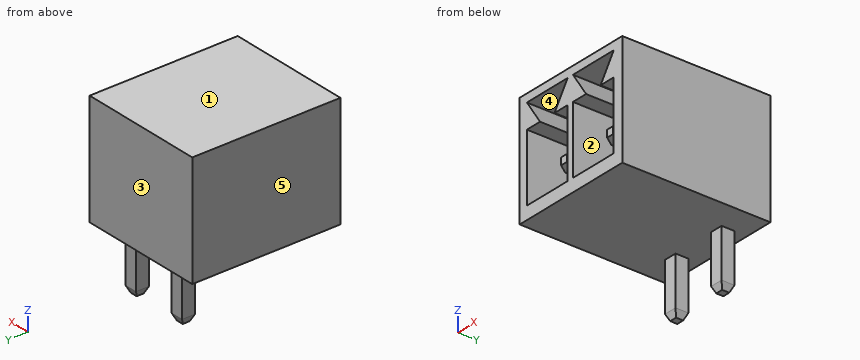
from build123d import *
from OCP.BRepFilletAPI import BRepFilletAPI_MakeChamfer

# Parameters (mm, degrees)
SKETCH_1_W                          = 7.8
SKETCH_1_H                          = 9.2
EXTRUDE_1_DEPTH                     = 7
SKETCH_2_W                          = 0.8
SKETCH_2_H                          = 0.8
EXTRUDE_2_DEPTH                     = 3.4
CHAMFER_1_SIZE                      = 0.4
CHAMFER_1_SIZE2                     = 0.178091474
CUT_EXTRUDE_1_DEPTH                 = 7
PATTERN_LINEAR_1_COUNT              = 3
PATTERN_LINEAR_1_PITCH              = 3.5
CHAMFER_1_OF_PATTERN_LINEAR_1_SIZE  = 0.4
CHAMFER_1_OF_PATTERN_LINEAR_1_SIZE2 = 0.178091474
PATTERN_LINEAR_2_COUNT              = 2
PATTERN_LINEAR_2_PITCH              = 3.5
SKETCH_4_W                          = 0.8
SKETCH_4_H                          = 0.8
EXTRUDE_3_DEPTH                     = 6
CHAMFER_2_SIZE                      = 0.4
CHAMFER_2_SIZE2                     = 0.178091474
PATTERN_LINEAR_3_COUNT              = 2
PATTERN_LINEAR_3_PITCH              = 3.5
CHAMFER_2_OF_PATTERN_LINEAR_3_SIZE  = 0.4
CHAMFER_2_OF_PATTERN_LINEAR_3_SIZE2 = 0.178091474


with BuildPart() as part:
    # Эскиз1 → Бобышка-Вытянуть1 (new body)
    with BuildSketch(Plane.XY):
        with Locations((0, 4.6)):
            Rectangle(SKETCH_1_W, SKETCH_1_H)
    extrude(amount=EXTRUDE_1_DEPTH)

    # Эскиз2 → Бобышка-Вытянуть2 (add)
    with BuildSketch(Plane(origin=(0, 0, 0), x_dir=(-1, 0, 0), z_dir=(0, 0, -1))):
        with Locations((-1.75, 8)):
            Rectangle(SKETCH_2_W, SKETCH_2_H)
    extrude_2 = extrude(amount=EXTRUDE_2_DEPTH)

    # Фаска1: one chamfer whose edges measure the first distance from different faces: ONE call of the kernel's chamfer builder (chamfer() names one face for all edges)
    chamfer_1_edges_1 = [part.edges().sort_by_distance(p)[0] for p in [
        (1.35, 8, -3.4),
    ]]
    chamfer_1_side_1 = [part.faces().sort_by_distance(p)[0] for p in [
        (1.35, 8, -1.7),
    ]]
    chamfer_1_edges_2 = [part.edges().sort_by_distance(p)[0] for p in [
        (1.75, 8.4, -3.4),
    ]]
    chamfer_1_side_2 = [part.faces().sort_by_distance(p)[0] for p in [
        (1.75, 8.4, -1.7),
    ]]
    chamfer_1_edges_3 = [part.edges().sort_by_distance(p)[0] for p in [
        (2.15, 8, -3.4),
    ]]
    chamfer_1_side_3 = [part.faces().sort_by_distance(p)[0] for p in [
        (2.15, 8, -1.7),
    ]]
    chamfer_1_edges_4 = [part.edges().sort_by_distance(p)[0] for p in [
        (1.75, 7.6, -3.4),
    ]]
    chamfer_1_side_4 = [part.faces().sort_by_distance(p)[0] for p in [
        (1.75, 7.6, -1.7),
    ]]
    chamfer_1 = BRepFilletAPI_MakeChamfer(part.part.solid().wrapped)
    for e in chamfer_1_edges_1:
        chamfer_1.Add(CHAMFER_1_SIZE, CHAMFER_1_SIZE2, e.wrapped, chamfer_1_side_1[0].wrapped)  # the first distance lies on this face
    for e in chamfer_1_edges_2:
        chamfer_1.Add(CHAMFER_1_SIZE, CHAMFER_1_SIZE2, e.wrapped, chamfer_1_side_2[0].wrapped)  # the first distance lies on this face
    for e in chamfer_1_edges_3:
        chamfer_1.Add(CHAMFER_1_SIZE, CHAMFER_1_SIZE2, e.wrapped, chamfer_1_side_3[0].wrapped)  # the first distance lies on this face
    for e in chamfer_1_edges_4:
        chamfer_1.Add(CHAMFER_1_SIZE, CHAMFER_1_SIZE2, e.wrapped, chamfer_1_side_4[0].wrapped)  # the first distance lies on this face
    add(Compound.cast(chamfer_1.Shape()), mode=Mode.REPLACE)

    # Эскиз3 → Вырез-Вытянуть1 (cut)
    with BuildSketch(Plane.XZ):
        Polygon((0.15, 0.8), (3.25, 0.8), (3.25, 5), (2.25, 5), (3.25, 6.5), (0.15, 6.5), (1.15, 5), (0.15, 5), align=None)
    cut_extrude_1 = extrude(amount=-CUT_EXTRUDE_1_DEPTH, mode=Mode.SUBTRACT)

    # Линейный массив1: Бобышка-Вытянуть2 ×3, 1 skipped
    with Locations(*[(-i * PATTERN_LINEAR_1_PITCH, 0, 0) for i in range(1, PATTERN_LINEAR_1_COUNT) if i not in (2,)]):
        add(extrude_2)

    # Фаска1 of Линейный массив1: one chamfer whose edges measure the first distance from different faces: ONE call of the kernel's chamfer builder (chamfer() names one face for all edges)
    chamfer_1_of_pattern_linear_1_edges_1 = [part.edges().sort_by_distance(p)[0] for p in [
        (-2.15, 8, -3.4),
    ]]
    chamfer_1_of_pattern_linear_1_side_1 = [part.faces().sort_by_distance(p)[0] for p in [
        (-2.15, 8, -1.7),
    ]]
    chamfer_1_of_pattern_linear_1_edges_2 = [part.edges().sort_by_distance(p)[0] for p in [
        (-1.75, 8.4, -3.4),
    ]]
    chamfer_1_of_pattern_linear_1_side_2 = [part.faces().sort_by_distance(p)[0] for p in [
        (-1.75, 8.4, -1.7),
    ]]
    chamfer_1_of_pattern_linear_1_edges_3 = [part.edges().sort_by_distance(p)[0] for p in [
        (-1.35, 8, -3.4),
    ]]
    chamfer_1_of_pattern_linear_1_side_3 = [part.faces().sort_by_distance(p)[0] for p in [
        (-1.35, 8, -1.7),
    ]]
    chamfer_1_of_pattern_linear_1_edges_4 = [part.edges().sort_by_distance(p)[0] for p in [
        (-1.75, 7.6, -3.4),
    ]]
    chamfer_1_of_pattern_linear_1_side_4 = [part.faces().sort_by_distance(p)[0] for p in [
        (-1.75, 7.6, -1.7),
    ]]
    chamfer_1_of_pattern_linear_1 = BRepFilletAPI_MakeChamfer(part.part.solid().wrapped)
    for e in chamfer_1_of_pattern_linear_1_edges_1:
        chamfer_1_of_pattern_linear_1.Add(CHAMFER_1_OF_PATTERN_LINEAR_1_SIZE, CHAMFER_1_OF_PATTERN_LINEAR_1_SIZE2, e.wrapped, chamfer_1_of_pattern_linear_1_side_1[0].wrapped)  # the first distance lies on this face
    for e in chamfer_1_of_pattern_linear_1_edges_2:
        chamfer_1_of_pattern_linear_1.Add(CHAMFER_1_OF_PATTERN_LINEAR_1_SIZE, CHAMFER_1_OF_PATTERN_LINEAR_1_SIZE2, e.wrapped, chamfer_1_of_pattern_linear_1_side_2[0].wrapped)  # the first distance lies on this face
    for e in chamfer_1_of_pattern_linear_1_edges_3:
        chamfer_1_of_pattern_linear_1.Add(CHAMFER_1_OF_PATTERN_LINEAR_1_SIZE, CHAMFER_1_OF_PATTERN_LINEAR_1_SIZE2, e.wrapped, chamfer_1_of_pattern_linear_1_side_3[0].wrapped)  # the first distance lies on this face
    for e in chamfer_1_of_pattern_linear_1_edges_4:
        chamfer_1_of_pattern_linear_1.Add(CHAMFER_1_OF_PATTERN_LINEAR_1_SIZE, CHAMFER_1_OF_PATTERN_LINEAR_1_SIZE2, e.wrapped, chamfer_1_of_pattern_linear_1_side_4[0].wrapped)  # the first distance lies on this face
    add(Compound.cast(chamfer_1_of_pattern_linear_1.Shape()), mode=Mode.REPLACE)

    # Линейный массив2: Вырез-Вытянуть1 ×2
    with Locations(*[(-i * PATTERN_LINEAR_2_PITCH, 0, 0) for i in range(1, PATTERN_LINEAR_2_COUNT)]):
        add(cut_extrude_1, mode=Mode.SUBTRACT)

    # Эскиз4 → Бобышка-Вытянуть3 (add)
    with BuildSketch(Plane.XZ.offset(-7)):
        with Locations((1.75, 3)):
            Rectangle(SKETCH_4_W, SKETCH_4_H)
    extrude_3 = extrude(amount=EXTRUDE_3_DEPTH)

    # Фаска2: one chamfer whose edges measure the first distance from different faces: ONE call of the kernel's chamfer builder (chamfer() names one face for all edges)
    chamfer_2_edges_1 = [part.edges().sort_by_distance(p)[0] for p in [
        (2.15, 1, 3),
    ]]
    chamfer_2_side_1 = [part.faces().sort_by_distance(p)[0] for p in [
        (2.15, 4, 3),
    ]]
    chamfer_2_edges_2 = [part.edges().sort_by_distance(p)[0] for p in [
        (1.75, 1, 3.4),
    ]]
    chamfer_2_side_2 = [part.faces().sort_by_distance(p)[0] for p in [
        (1.75, 4, 3.4),
    ]]
    chamfer_2_edges_3 = [part.edges().sort_by_distance(p)[0] for p in [
        (1.35, 1, 3),
    ]]
    chamfer_2_side_3 = [part.faces().sort_by_distance(p)[0] for p in [
        (1.35, 4, 3),
    ]]
    chamfer_2_edges_4 = [part.edges().sort_by_distance(p)[0] for p in [
        (1.75, 1, 2.6),
    ]]
    chamfer_2_side_4 = [part.faces().sort_by_distance(p)[0] for p in [
        (1.75, 4, 2.6),
    ]]
    chamfer_2 = BRepFilletAPI_MakeChamfer(part.part.solid().wrapped)
    for e in chamfer_2_edges_1:
        chamfer_2.Add(CHAMFER_2_SIZE, CHAMFER_2_SIZE2, e.wrapped, chamfer_2_side_1[0].wrapped)  # the first distance lies on this face
    for e in chamfer_2_edges_2:
        chamfer_2.Add(CHAMFER_2_SIZE, CHAMFER_2_SIZE2, e.wrapped, chamfer_2_side_2[0].wrapped)  # the first distance lies on this face
    for e in chamfer_2_edges_3:
        chamfer_2.Add(CHAMFER_2_SIZE, CHAMFER_2_SIZE2, e.wrapped, chamfer_2_side_3[0].wrapped)  # the first distance lies on this face
    for e in chamfer_2_edges_4:
        chamfer_2.Add(CHAMFER_2_SIZE, CHAMFER_2_SIZE2, e.wrapped, chamfer_2_side_4[0].wrapped)  # the first distance lies on this face
    add(Compound.cast(chamfer_2.Shape()), mode=Mode.REPLACE)

    # Линейный массив3: Бобышка-Вытянуть3 ×2
    with Locations(*[(-i * PATTERN_LINEAR_3_PITCH, 0, 0) for i in range(1, PATTERN_LINEAR_3_COUNT)]):
        add(extrude_3)

    # Фаска2 of Линейный массив3: one chamfer whose edges measure the first distance from different faces: ONE call of the kernel's chamfer builder (chamfer() names one face for all edges)
    chamfer_2_of_pattern_linear_3_edges_1 = [part.edges().sort_by_distance(p)[0] for p in [
        (-1.35, 1, 3),
    ]]
    chamfer_2_of_pattern_linear_3_side_1 = [part.faces().sort_by_distance(p)[0] for p in [
        (-1.35, 4, 3),
    ]]
    chamfer_2_of_pattern_linear_3_edges_2 = [part.edges().sort_by_distance(p)[0] for p in [
        (-1.75, 1, 3.4),
    ]]
    chamfer_2_of_pattern_linear_3_side_2 = [part.faces().sort_by_distance(p)[0] for p in [
        (-1.75, 4, 3.4),
    ]]
    chamfer_2_of_pattern_linear_3_edges_3 = [part.edges().sort_by_distance(p)[0] for p in [
        (-2.15, 1, 3),
    ]]
    chamfer_2_of_pattern_linear_3_side_3 = [part.faces().sort_by_distance(p)[0] for p in [
        (-2.15, 4, 3),
    ]]
    chamfer_2_of_pattern_linear_3_edges_4 = [part.edges().sort_by_distance(p)[0] for p in [
        (-1.75, 1, 2.6),
    ]]
    chamfer_2_of_pattern_linear_3_side_4 = [part.faces().sort_by_distance(p)[0] for p in [
        (-1.75, 4, 2.6),
    ]]
    chamfer_2_of_pattern_linear_3 = BRepFilletAPI_MakeChamfer(part.part.solid().wrapped)
    for e in chamfer_2_of_pattern_linear_3_edges_1:
        chamfer_2_of_pattern_linear_3.Add(CHAMFER_2_OF_PATTERN_LINEAR_3_SIZE, CHAMFER_2_OF_PATTERN_LINEAR_3_SIZE2, e.wrapped, chamfer_2_of_pattern_linear_3_side_1[0].wrapped)  # the first distance lies on this face
    for e in chamfer_2_of_pattern_linear_3_edges_2:
        chamfer_2_of_pattern_linear_3.Add(CHAMFER_2_OF_PATTERN_LINEAR_3_SIZE, CHAMFER_2_OF_PATTERN_LINEAR_3_SIZE2, e.wrapped, chamfer_2_of_pattern_linear_3_side_2[0].wrapped)  # the first distance lies on this face
    for e in chamfer_2_of_pattern_linear_3_edges_3:
        chamfer_2_of_pattern_linear_3.Add(CHAMFER_2_OF_PATTERN_LINEAR_3_SIZE, CHAMFER_2_OF_PATTERN_LINEAR_3_SIZE2, e.wrapped, chamfer_2_of_pattern_linear_3_side_3[0].wrapped)  # the first distance lies on this face
    for e in chamfer_2_of_pattern_linear_3_edges_4:
        chamfer_2_of_pattern_linear_3.Add(CHAMFER_2_OF_PATTERN_LINEAR_3_SIZE, CHAMFER_2_OF_PATTERN_LINEAR_3_SIZE2, e.wrapped, chamfer_2_of_pattern_linear_3_side_4[0].wrapped)  # the first distance lies on this face
    add(Compound.cast(chamfer_2_of_pattern_linear_3.Shape()), mode=Mode.REPLACE)


solid = part.part
Can you work these out from the model? Positions are in its coordinate system, mm. Face numbers are marked on the shaded views. A direction names the side the tool comes from. Coordinates: 2 decimals unless noted, no trailing zeros. Write each loop counter-clockwise with the first axis right and the second up, starting at its lowest first coordinate (ties: lowest second). Pieces come first, ordered by that corner, then holes. Notation, with made-up numbers: (56, 29.5) - (66, 29.5) arc R11 ccw to (66, 35.5) - close; hole circle Ø3 at (-27, 71.25). An arc over 180 degrees is marked (long way). Return JSON: item names as keys, results as strings. Group by question number.
Item 1: If we section it at A-A (y = 5.5): Write out the boundary of the cut face in (x, z), then the cut area to 3 significant figures.
Item 2: If we section it at C-C (x = -2.75): Write out the boundary of the cut face in (y, z), then the cut area to 3 significant figures.
Item 3: Which directions (+Z, -Z, +X, -X, +Y, -Y) give clear straight access to the entire face, cutting with the end or side of a thin tool? Please do the marked faces 4 and 5.
Item 4: Please list where these lines run through material, in increasing order: probe 1 along X at (y, z) = (4, 4.5); probe 2 along Z at (x, y) = (2, 5); probe 3 along X at (y, z) = (2, 5.5).
Item 5: If we section it at D-D (z = 1): Write out the boundary of the cut face in (x, y).
Item 6: We'd pull the mould along Z, two halves only. Please class the marked faces 1, 2 and 3: pulls with the +Z half, pulls with the -Z half, needs draft (parallel to the pull), parting line crosses it, or undercut.
Item 7: If we section it at B-B (z = -0.5): Write out the boundary of the cut face in (x, y), then the cut area to 3 significant figures.
Item 8: I'm going to push flat-ended pins straight in: pin 1 Ø0.6 at (x, y) = (-1.5, 3) entering from -Z; pin 2 Ø0.6 at (y, z) = (8, -2) entering from -X; pin 3 Ø0.5 at (x, z) = (1.5, 3) entering from -Y. Where does each tip first touch, or does it pass through?
Return value:
{
 "1": {"outline": "(-3.9, 0) - (3.9, 0) - (3.9, 7) - (-3.9, 7) - close; (-2.15, 2.6) - (-1.35, 2.6) - (-1.35, 3.4) - (-2.15, 3.4) - close; (1.35, 2.6) - (2.15, 2.6) - (2.15, 3.4) - (1.35, 3.4) - close; hole (-3.35, 0.8) - (-0.25, 0.8) - (-0.25, 5) - (-1.25, 5) - (-0.25, 6.5) - (-3.35, 6.5) - (-2.35, 5) - (-3.35, 5) - close; hole (0.15, 0.8) - (3.25, 0.8) - (3.25, 5) - (2.25, 5) - (3.25, 6.5) - (0.15, 6.5) - (1.15, 5) - (0.15, 5) - close", "area": "23.5 mm^2"},
 "2": {"outline": "(0, 0) - (9.2, 0) - (9.2, 7) - (0, 7) - (0, 6.5) - (7, 6.5) - (7, 5.6) - (0, 5.6) - (0, 5) - (7, 5) - (7, 0.8) - (0, 0.8) - close", "area": "28.7 mm^2"},
 "3": {"face 4": "-Y", "face 5": "+Z, -Z, -X, +Y, -Y"},
 "4": {"probe 1": "x = -3.9 to -3.35, -0.25 to 0.15, 3.25 to 3.9", "probe 2": "z = 0 to 0.8, 2.6 to 3.4, 6.5 to 7", "probe 3": "x = -3.9 to -2.68, -0.92 to 0.82, 2.58 to 3.9"},
 "5": {"outline": "(-3.9, 0) - (-3.35, 0) - (-3.35, 7) - (-0.25, 7) - (-0.25, 0) - (0.15, 0) - (0.15, 7) - (3.25, 7) - (3.25, 0) - (3.9, 0) - (3.9, 9.2) - (-3.9, 9.2) - close"},
 "6": {"face 1": "pulls with the +Z half", "face 2": "undercut", "face 3": "needs draft"},
 "7": {"outline": "(-2.15, 7.6) - (-1.35, 7.6) - (-1.35, 8.4) - (-2.15, 8.4) - close; (1.35, 7.6) - (2.15, 7.6) - (2.15, 8.4) - (1.35, 8.4) - close", "area": "1.28 mm^2"},
 "8": {"pin 1": "stops at z = 0", "pin 2": "stops at x = -2.15", "pin 3": "stops at y = 1"}
}
